Work out the finished part from the listing and answer in its coordinate system (mm). Give positions to 0.01 mm unless a question says otherwise; leave off trailing zeros. Loops run counter-clockwise (first coordinate to the right, second up) from the corner with the lowest first, then second, coordinate; pieces in that order, holes last. Notation, with made-up numbers: (-26.5, 10.25) - (-6.5, 10.25) arc R14 cw to (-6.5, 16.25) - close; hole circle Ø7 at (44, 10.25). An arc over 180 degrees is marked (long way). Use one line per item in the form item = value. Start each with the question number.
from build123d import *

# Parameters (mm, degrees)
SKETCH_2_R               = 0.2
EXTRUDE_1_DEPTH          = 5
PATTERN_CIRCULAR_1_COUNT = 9


with BuildPart() as part:
    # 草图1 → 旋转1 (revolve)
    with BuildSketch(Plane.XY):
        with BuildLine():
            Line((-3.6, 71), (-3.6, 0))
            Line((-3.6, 0), (0, 0))
            Line((0, 0), (0, 78))
            add(Edge.make_bspline(
                [(-3.6, 71), (-3.337937783, 73.551680107), (-2.931620403, 77.076293538), (0, 78)],
                knots=[0, 0, 0, 0, 1, 1, 1, 1], degree=3))
        make_face()
    revolve(axis=Axis((0, 8.263328558, 0), (0, -1, 0)))

    # 草图2 → 凸台-拉伸1 (add)
    with BuildSketch(Plane.XZ):
        with Locations((-0.987826351, -1.383545843)):
            Circle(SKETCH_2_R)
    extrude_1 = extrude(amount=EXTRUDE_1_DEPTH)

    # 阵列(圆周)1: 凸台-拉伸1 ×9 about axis
    pattern_circular_1_axis = Axis((0, 0, 0), (0, 1, 0))
    for i in range(1, PATTERN_CIRCULAR_1_COUNT):
        add(extrude_1.rotate(pattern_circular_1_axis, i * 360 / PATTERN_CIRCULAR_1_COUNT))


solid = part.part
1) Find the intervals of material crossed by probe 1 along Z at (x, y) = (-2.75, 37.5); probe 2 along Z at (x, y) = (2.25, 69.5); probe 3 along X at (y, z) = (4, 0.5), in increasing order.
2) A cutting plane is placed at A-A (y = 57.5). Give the vertices of the cut face in (x, z), plus the area to 3 significant figures.
3) Determine the mould class of faces 1 (the cylindrical face through (-3.434, 35.003, -1.081)), 2 (the flat face through (0, 0, 0)) for opening direction Y: released by +Y, released by -Y, zero draft, split by the parting line, or undercut.
4) Flat-ended cylindrical pins translate along their axes: pin 1 Ø1 at (y, z) = (68.5, 1.5) entering from -X; pin 2 Ø1.5 at (x, y) = (-2, 22) entering from +Z; pin 3 Ø3 at (x, z) = (-2, 2) entering from +Y. Find the tip coordinate at first contact, or state that the pin passes through.
Answer sheet:
q1.probe_1 = -2.32 to 2.32
q1.probe_2 = -2.81 to 2.81
q1.probe_3 = -3.57 to 3.57
q2.outline = circle Ø7.2 at (0, 0)
q2.area = 40.7 mm²
q3.face_1 = zero draft
q3.face_2 = released by -Y
q4.pin_1 = -3.46
q4.pin_2 = 3.38
q4.pin_3 = 77.29
